```python
from build123d import *

# Parameters (mm, degrees)
SKETCH1_W           = 60.4
SKETCH1_H           = 33.4
SKETCH1_W_2         = 58.4
SKETCH1_H_2         = 31.4
BOSS_EXTRUDE1_DEPTH = 19
SKETCH2_W           = 60.4
SKETCH2_H           = 33.4
SKETCH2_W_2         = 20.2
SKETCH2_H_2         = 15.2
BOSS_EXTRUDE2_DEPTH = 1
SKETCH3_R           = 1.25
BOSS_EXTRUDE3_DEPTH = 14
CUT_EXTRUDE1_REACH  = 67.78
SKETCH4_W           = 8
SKETCH4_H           = 4


with BuildPart() as part:
    # Sketch1 → Boss-Extrude1 (new body)
    with BuildSketch(Plane(origin=(0, 0, 0), x_dir=(1, 0, 0), z_dir=(0, 1, 0))):
        Rectangle(SKETCH1_W, SKETCH1_H)
        Rectangle(SKETCH1_W_2, SKETCH1_H_2, mode=Mode.SUBTRACT)
    extrude(amount=BOSS_EXTRUDE1_DEPTH)

    # Sketch2 → Boss-Extrude2 (add)
    with BuildSketch(Plane(origin=(0, 19, 0), x_dir=(1, 0, 0), z_dir=(0, 1, 0))):
        Rectangle(SKETCH2_W, SKETCH2_H)
        Rectangle(SKETCH2_W_2, SKETCH2_H_2, mode=Mode.SUBTRACT)
    extrude(amount=BOSS_EXTRUDE2_DEPTH)

    # Sketch3 → Boss-Extrude3 (add)
    # profile 1 of 4: a face of its own
    with BuildSketch(Plane.XZ.offset(-19)):
        with BuildLine():
            Line((-29.2, 15.7), (-26, 15.7))
            Line((-26, 15.7), (-26, 15.592329219))
            ThreePointArc((-26, 15.592329219), (-25.80860754, 15.003980814), (-25.307692308, 14.640843306))
            ThreePointArc((-25.307692308, 14.640843306), (-24.409009742, 10.909009742), (-28.140843306, 11.807692308))
            ThreePointArc((-28.140843306, 11.807692308), (-28.503980814, 12.30860754), (-29.092329219, 12.5))
            Line((-29.092329219, 12.5), (-29.2, 12.5))
            Line((-29.2, 12.5), (-29.2, 15.7))
        make_face()
        with Locations(Location((-26, 12.5, 0), (0, 0, 90))):
            Circle(SKETCH3_R, mode=Mode.SUBTRACT)
    # profile 2 of 4: a face of its own
    with BuildSketch(Plane.XZ.offset(-19)):
        with BuildLine():
            Line((29.2, 12.5), (29.2, 15.7))
            Line((29.2, 15.7), (26, 15.7))
            Line((26, 15.7), (26, 15.592329219))
            ThreePointArc((26, 15.592329219), (25.80860754, 15.003980814), (25.307692308, 14.640843306))
            ThreePointArc((25.307692308, 14.640843306), (24.409009742, 10.909009742), (28.140843306, 11.807692308))
            ThreePointArc((28.140843306, 11.807692308), (28.503980814, 12.30860754), (29.092329219, 12.5))
            Line((29.092329219, 12.5), (29.2, 12.5))
        make_face()
        with Locations(Location((26, 12.5, 0), (0, 0, 90))):
            Circle(SKETCH3_R, mode=Mode.SUBTRACT)
    # profile 3 of 4: a face of its own
    with BuildSketch(Plane.XZ.offset(-19)):
        with BuildLine():
            Line((29.2, -15.7), (26, -15.7))
            Line((26, -15.7), (26, -15.592329219))
            ThreePointArc((26, -15.592329219), (25.80860754, -15.003980814), (25.307692308, -14.640843306))
            ThreePointArc((25.307692308, -14.640843306), (24.409009742, -10.909009742), (28.140843306, -11.807692308))
            ThreePointArc((28.140843306, -11.807692308), (28.503980814, -12.30860754), (29.092329219, -12.5))
            Line((29.092329219, -12.5), (29.2, -12.5))
            Line((29.2, -12.5), (29.2, -15.7))
        make_face()
        with Locations(Location((26, -12.5, 0), (0, 0, 90))):
            Circle(SKETCH3_R, mode=Mode.SUBTRACT)
    # profile 4 of 4: a face of its own
    with BuildSketch(Plane.XZ.offset(-19)):
        with BuildLine():
            Line((-29.2, -12.5), (-29.2, -15.7))
            Line((-29.2, -15.7), (-26, -15.7))
            Line((-26, -15.7), (-26, -15.592329219))
            ThreePointArc((-26, -15.592329219), (-25.80860754, -15.003980814), (-25.307692308, -14.640843306))
            ThreePointArc((-25.307692308, -14.640843306), (-24.409009742, -10.909009742), (-28.140843306, -11.807692308))
            ThreePointArc((-28.140843306, -11.807692308), (-28.503980814, -12.30860754), (-29.092329219, -12.5))
            Line((-29.092329219, -12.5), (-29.2, -12.5))
        make_face()
        with Locations(Location((-26, -12.5, 0), (0, 0, 90))):
            Circle(SKETCH3_R, mode=Mode.SUBTRACT)
    extrude(amount=BOSS_EXTRUDE3_DEPTH)

    # Sketch4 → Cut-Extrude1 (cut, up to next)
    with BuildSketch(Plane.ZY.offset(30.2), mode=Mode.PRIVATE) as cut_extrude1_sk1:
        with Locations((0, 2)):
            Rectangle(SKETCH4_W, SKETCH4_H)
    cut_extrude1_tool1 = extrude(cut_extrude1_sk1.sketch, amount=-CUT_EXTRUDE1_REACH, mode=Mode.PRIVATE) & part.part
    add(cut_extrude1_tool1.solids().sort_by_distance((-30.2, 2, 0))[0], mode=Mode.SUBTRACT)


solid = part.part
```
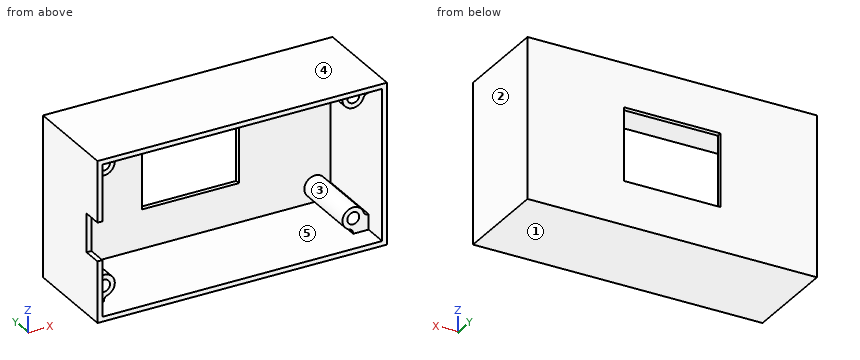
Input: part model. Units: mm. Frame: model coordinates. Face numbers are marked on the shaded views. A direction names the side the tool comes from. Coordinates: 2 decimals unless noted, no trailing zeros. Write each loop counter-clockwise with the first axis right and the second up, starting at its lowest first coordinate (ties: lowest second). Pieces come first, ordered by that corner, then holes.
1) Set-up query: the marked faces 4 and 5. Return all of +Z, -Z, +X, -X, +Y, -Y with unobstructed straight access to the full face (end or side cutting, diameter ignored); none if empty.
2) Section D-D on x = 12. Output: boundary loops of the cut face in (y, z), and give its area (3 significant figures).
3) Section B-B on y = 6. State how many separate pieces and enclosed holes the cut face has, and give its area (3 significant figures).
4) Section A-A on x = 3.5. Output: boundary loops of the cut face in (y, z).
5) Mould query, pull axis X, two halves, no side actions, for the marked faces 1, 2 and 3. Classes: pulls with the +X half, pulls with the -X half, needs draft (parallel to the pull), parting line crosses it, or undercut.
6) Section C-C on z = -9. Output: boundary loops of the cut face in (x, y).
7) Pin query (flat end, axial travel): pin 1 Ø3 at (x, z) = (25.5, 12.5) entering from -Y; pin 2 Ø0.8 at (x, z) = (25.5, -12.5) entering from -Y; pin 3 Ø0.5 at (x, z) = (-30, 0) entering from -Y. Return the tip coordinate at first contact, or that it passes through.
8) Material intervals for line 1 along Z through (x, y) = (13, 6.5); line 2 along X through (y, z) = (6.5, -7); line 3 along X through (y, z) = (10.5, 11.5), sorted ascending.
Check result:
1. face 4: +Z, +X, -X, +Y, -Y
1. face 5: -Y
2. outline: (0, -16.7) - (20, -16.7) - (20, 16.7) - (0, 16.7) - (0, 15.7) - (19, 15.7) - (19, -15.7) - (0, -15.7) - close
2. area: 71.4 mm2
3. separate pieces: 1
3. enclosed holes: 5
3. area: 254 mm2
4. outline: (0, -16.7) - (20, -16.7) - (20, -7.6) - (19, -7.6) - (19, -15.7) - (0, -15.7) - close; (0, 15.7) - (19, 15.7) - (19, 7.6) - (20, 7.6) - (20, 16.7) - (0, 16.7) - close
5. face 1: needs draft
5. face 2: pulls with the +X half
5. face 3: undercut
6. outline: (-30.2, 0) - (-29.2, 0) - (-29.2, 19) - (29.2, 19) - (29.2, 0) - (30.2, 0) - (30.2, 20) - (-30.2, 20) - close
7. pin 1: stops at y = 5
7. pin 2: stops at y = 19
7. pin 3: stops at y = 4
8. line 1: z = -16.7 to -15.7, 15.7 to 16.7
8. line 2: x = -30.2 to -29.2, 29.2 to 30.2
8. line 3: x = -30.2 to -29.2, -28.02 to -26.75, -25.25 to -23.98, 23.98 to 25.25, 26.75 to 28.02, 29.2 to 30.2
